Source: three-view drawing plus pictorial views. Frame: mm from the lowest corner of the part. Give positions to 0.01 mm unless a question says otherwise; leave off trailing zeros. Loops run counter-clockwise (first coordinate to the right, second up) from the corner with the lowest first, then second, coordinate; pieces in that order, holes last. Notation, with made-up numbers: M -16,-15 L 13,-15 A22 ccw 13,-4 Z; hole C 43.5,21.5 d11. An arc over 180 degrees is marked long. Write item = value, one per line.
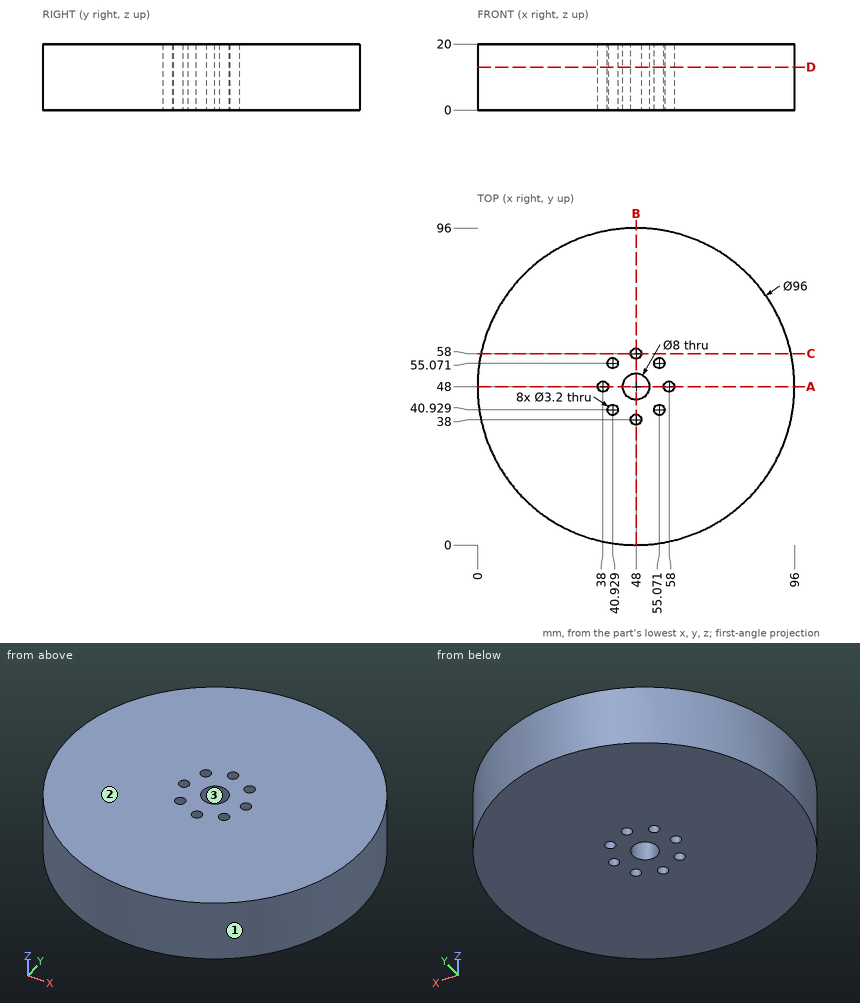
1. Cut plane D-D, the plane z = 13. Count the separate pieces of the cut face and the enclosed holes in it, then the cut area to 3 significant figures.
Derived:
separate_pieces = 1
enclosed_holes = 9
area = 7,120 mm²
2. First-contact query: pin 1 Ø1.5 at (y, z) = (63.5, 11) entering from +X; pin 2 Ø1 at (x, z) = (63.5, 8.5) entering from +Y; pin 3 Ø3 at (y, z) = (30, 3) entering from +X (3 decimals). Flat tips, straight axial feed; report the tip coordinate or a pass-through.
Derived:
pin_1 = 93.68
pin_2 = 93.6
pin_3 = 93.075
3. Material intervals for probe 1 along Y at (x, z) = (48, 8.75); probe 2 along X at (y, z) = (12, 2.5); probe 3 along Y at (x, z) = (23.5, 6.75), sorted ascending. Write a range as from..to.
Derived:
probe_1 = 0..36.4, 39.6..44, 52..56.4, 59.6..96
probe_2 = 16.25..79.75
probe_3 = 6.72..89.28
4. Cut plane A-A, the plane y = 48. Return the cut outline in (x, z), then the cut area to 3 significant figures.
Derived:
outline = M 0,0 L 36.4,0 L 36.4,20 L 0,20 Z; M 39.6,0 L 44,0 L 44,20 L 39.6,20 Z; M 52,0 L 56.4,0 L 56.4,20 L 52,20 Z; M 59.6,0 L 96,0 L 96,20 L 59.6,20 Z
area = 1,630 mm²
5. Pull-direction query (Y, two-part tool) for the marked faces 1, 2 and 3; classes: +Y half, -Y half, draft (parallel to the pull), parting line (faces both ways), or undercut.
Derived:
face_1 = parting line
face_2 = draft
face_3 = undercut
6. Cut plane C-C, the plane y = 58. Return the cut outline in (x, z), then the cut area to 3 significant figures.
Derived:
outline = M 1.05,0 L 46.4,0 L 46.4,20 L 1.05,20 Z; M 49.6,0 L 94.95,0 L 94.95,20 L 49.6,20 Z
area = 1,810 mm²
